from build123d import *

# Parameters (mm, degrees)
SKETCH1_W                = 22.5
SKETCH1_H                = 7
BOSS_EXTRUDE1_DEPTH      = 1.5
SKETCH2_R                = 1.475
BOSS_EXTRUDE2_DEPTH      = 13.5
SKETCH3_R                = 1.05
BOSS_EXTRUDE3_DEPTH      = 10.5
SKETCH4_W                = 22.5
SKETCH4_H                = 2.5
SKETCH4_H_2              = 7
BOSS_EXTRUDE4_DEPTH      = 6
BOSS_EXTRUDE4_DEPTH_BACK = 1.5
SKETCH5_W                = 3
SKETCH5_H                = 10
BOSS_EXTRUDE6_DEPTH      = 5
SKETCH7_W                = 11.5
SKETCH7_H                = 2
CUT_EXTRUDE1_DEPTH       = 7.5
SKETCH8_W                = 22.5
SKETCH8_H                = 9.5
BOSS_EXTRUDE7_DEPTH      = 2.61
SKETCH9_R                = 2.4
BOSS_EXTRUDE8_DEPTH      = 7.76
BOSS_EXTRUDE8_DEPTH_BACK = 1.5


with BuildPart() as part:
    # Sketch1 → Boss-Extrude1 (new body)
    with BuildSketch(Plane(origin=(0, 0, 0), x_dir=(1, 0, 0), z_dir=(0, 1, 0))):
        with Locations((-28.93578967, -21.079480712)):
            Rectangle(SKETCH1_W, SKETCH1_H)
    extrude(amount=BOSS_EXTRUDE1_DEPTH)

    # Sketch2 → Boss-Extrude2 (add)
    with BuildSketch(Plane(origin=(0, 1.5, 0), x_dir=(1, 0, 0), z_dir=(0, 1, 0))):
        with Locations((-37.53578967, -19.579480712)):
            Circle(SKETCH2_R)
        with Locations((-20.33578967, -19.579480712)):
            Circle(SKETCH2_R)
    extrude(amount=BOSS_EXTRUDE2_DEPTH)

    # Sketch3 → Boss-Extrude3 (add)
    with BuildSketch(Plane(origin=(0, 1.5, 0), x_dir=(1, 0, 0), z_dir=(0, 1, 0))):
        with Locations((-37.88578967, -23.029480712)):
            Circle(SKETCH3_R)
        with Locations((-19.98578967, -23.029480712)):
            Circle(SKETCH3_R)
    extrude(amount=BOSS_EXTRUDE3_DEPTH)

    # Sketch4 → Boss-Extrude4 (add, two sides)
    with BuildSketch(Plane(origin=(0, 0, 0), x_dir=(-1, 0, 0), z_dir=(0, -1, 0))) as boss_extrude4_sk:
        with Locations((28.93578967, -25.829480712)):
            Rectangle(SKETCH4_W, SKETCH4_H)
        with Locations((28.93578967, -21.079480712)):
            Rectangle(SKETCH4_W, SKETCH4_H_2)
    extrude(amount=BOSS_EXTRUDE4_DEPTH)
    extrude(boss_extrude4_sk.sketch, amount=-BOSS_EXTRUDE4_DEPTH_BACK)

    # Sketch5 → Boss-Extrude6 (add)
    with BuildSketch(Plane(origin=(0, -6, 0), x_dir=(-1, 0, 0), z_dir=(0, -1, 0))):
        with Locations((33.93578967, -32.079480712)):
            Rectangle(SKETCH5_W, SKETCH5_H)
        with Locations((22.43578967, -32.079480712)):
            Rectangle(SKETCH5_W, SKETCH5_H)
    extrude(amount=-BOSS_EXTRUDE6_DEPTH)

    # Sketch7 → Cut-Extrude1 (cut)
    with BuildSketch(Plane.XY.offset(37.079480712)):
        with Locations((-28.18578967, -3.5)):
            Rectangle(SKETCH7_W, SKETCH7_H)
    extrude(amount=-CUT_EXTRUDE1_DEPTH, mode=Mode.SUBTRACT)

    # Sketch8 → Boss-Extrude7 (add)
    with BuildSketch(Plane(origin=(0, 1.5, 0), x_dir=(1, 0, 0), z_dir=(0, 1, 0))):
        with Locations((-28.93578967, -22.329480712)):
            Rectangle(SKETCH8_W, SKETCH8_H)
    extrude(amount=BOSS_EXTRUDE7_DEPTH)

    # Sketch9 → Boss-Extrude8 (add, two sides)
    with BuildSketch(Plane(origin=(0, -6, 0), x_dir=(-1, 0, 0), z_dir=(0, -1, 0))) as boss_extrude8_sk:
        with Locations((28.81078967, -25.489480712)):
            Circle(SKETCH9_R)
        with Locations((28.81078967, -17.519480712)):
            Circle(SKETCH9_R)
    extrude(amount=BOSS_EXTRUDE8_DEPTH)
    extrude(boss_extrude8_sk.sketch, amount=-BOSS_EXTRUDE8_DEPTH_BACK)


solid = part.part
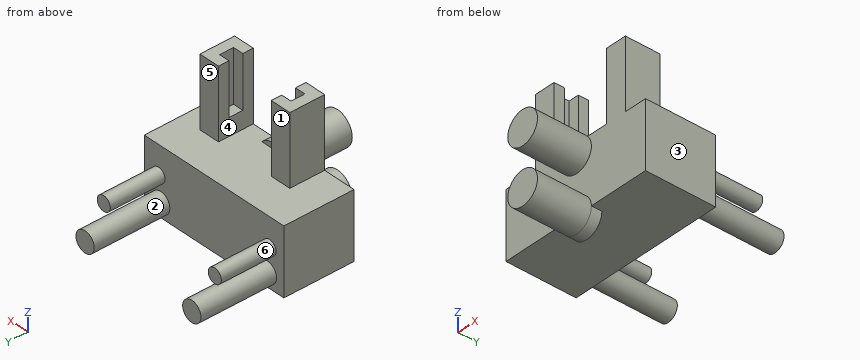
Source: CAD feature listing. Evaluate the final solid. Frame: model axes, mm. Face numbers are marked on the shaded views. A direction names the side the tool comes from. Coordinates: 2 decimals unless noted, no trailing zeros. Loops run counter-clockwise (first coordinate to the right, second up) from the corner with the lowest first, then second, coordinate; pieces in that order, holes last. Notation, with made-up numbers: (63, -25) - (79, -25) arc R19 cw to (79, -16) - close; hole circle Ø3 at (86.25, 49.25). An arc over 180 degrees is marked (long way). Return JSON: item names as keys, results as strings.
Q1. Material intervals for line 1 along Y through (x, z) = (-22.75, 32); line 2 along X through (y, z) = (-5.5, 34.75); line 3 along Y through (x, z) = (-35, 29), sorted ascending.
Results:
{"line 1": "-6 to -4.5, -2.5 to -1", "line 2": "-35.44 to -32.44, -23.94 to -20.94", "line 3": "-6 to -1"}
Q2. Access query for the marked faces 4, 5 and 6. Directions: +Z, -Z, +X, -X, +Y, -Y. A direction counts if a zero-diameter tool reaches every point of the face in a straight line with its end or side. Return the directions, or none.
Results:
{"face 4": "+Z, +Y, -Y", "face 5": "+Z, +X, -X, +Y", "face 6": "+Y"}
Q3. Section D-D, the plane x = -28.5. Return loops of the section in (y, z).
Results:
{"outline": "(-13.76, 15.14) - (-4.5, 15.14) - (-4.5, 17.58) - (4.11, 17.58) - (4.11, 27.08) - (-4.5, 27.08) - (-4.5, 27.87) - (-13.76, 27.87) - (-13.76, 23.11) - (-6, 23.11) - (-6, 19.9) - (-13.76, 19.9) - close"}
Q4. Section B-B, the plane y = -8.75. Return loops of the section in (x, z), plus the area to 3 significant figures.
Results:
{"outline": "circle Ø4.8 at (-28.81, 17.52); circle Ø4.8 at (-28.81, 25.49)", "area": "36.2 mm2"}
Q5. Mould query, pull axis X, two halves, no side actions, for the marked faces 1, 2 and 3. Classes: released by +X, released by -X, zero draft, split by the parting line, or undercut.
Results:
{"face 1": "zero draft", "face 2": "undercut", "face 3": "released by +X"}
Q6. Contact query for flat-ended pins moving along their axis: P1, Ø6, axis at x = -29, z = 27, coming from the +Y side; P2, Ø4, axis at x = -33, y = 3, coming from the +Z side; P3, Ø3, axis at x = -21.5, y = 10, coming from the +Z side. Output: stop coordinate, or through.
Results:
{"P1": "y = 4.11", "P2": "z = 27.08", "P3": "z = 24.08"}
Q7. Section A-A, the plane z = 31.25. Return loops of the section in (x, y), plus the area to 3 significant figures.
Results:
{"outline": "(-35.44, -6) - (-32.44, -6) - (-32.44, -4.5) - (-33.94, -4.5) - (-33.94, -2.5) - (-32.44, -2.5) - (-32.44, -1) - (-35.44, -1) - close; (-23.94, -6) - (-20.94, -6) - (-20.94, -1) - (-23.94, -1) - (-23.94, -2.5) - (-22.44, -2.5) - (-22.44, -4.5) - (-23.94, -4.5) - close", "area": "24.0 mm2"}
Q8. Section C-C, the plane z = 19. Return loops of the section in (x, y).
Results:
{"outline": "(-40.19, -6) - (-30.7, -6) - (-30.7, -13.76) - (-26.92, -13.76) - (-26.92, -6) - (-17.69, -6) - (-17.69, 4.11) - (-18.98, 4.11) - (-18.98, 15) - (-21.69, 15) - (-21.69, 4.11) - (-36.18, 4.11) - (-36.18, 15) - (-38.89, 15) - (-38.89, 4.11) - (-40.19, 4.11) - close"}
